For this review, use the dimensioned drawing (mm, ordinates from the lowest corner) and the shaded views. Round coordinates to 2 decimals unless told otherwise and drop trailing zeros. Loops run counter-clockwise (first coordinate to the right, second up) from the corner with the lowest first, then second, coordinate; pieces in that order, holes last. Notation, with made-up numbers: (68.5, 2) -> (108.5, 2) arc R25 ccw to (108.5, 24) -> close; hole circle Ø8 at (9.5, -25). An arc over 180 degrees is marked (long way). Answer as CSV lines item,"result". Start each with the question number.
(1) Draft analysis for pull direction X (two halves, no side actions). For the marked faces 1, 2 and 3, state which applies: +X half, -X half, draft (parallel to the pull), parting line (faces both ways), or undercut.
(2) Take a section at C-C, the plane x = 52. Write out the cut boundary in (y, z), and give its area (3 significant figures).
(3) For P1, Ø15, axis at y = 7.5, z = 29, coming from the -X side; P2, Ø2, axis at x = 76, z = 15.5, coming from the -Y side; P3, Ø15, axis at y = 13.5, z = 31, coming from the +X side, all flat-tipped, find the tip position at first contact; note any pin that passes through.
(4) Take a section at A-A, the plane y = 9. Write out the cut boundary in (x, z).
(5) To check wall thickness, follow line 1 (Y direction, x = 48, z = 57). State the ranges of the line that lie inside material, in increasing order. Write a range as from..to.
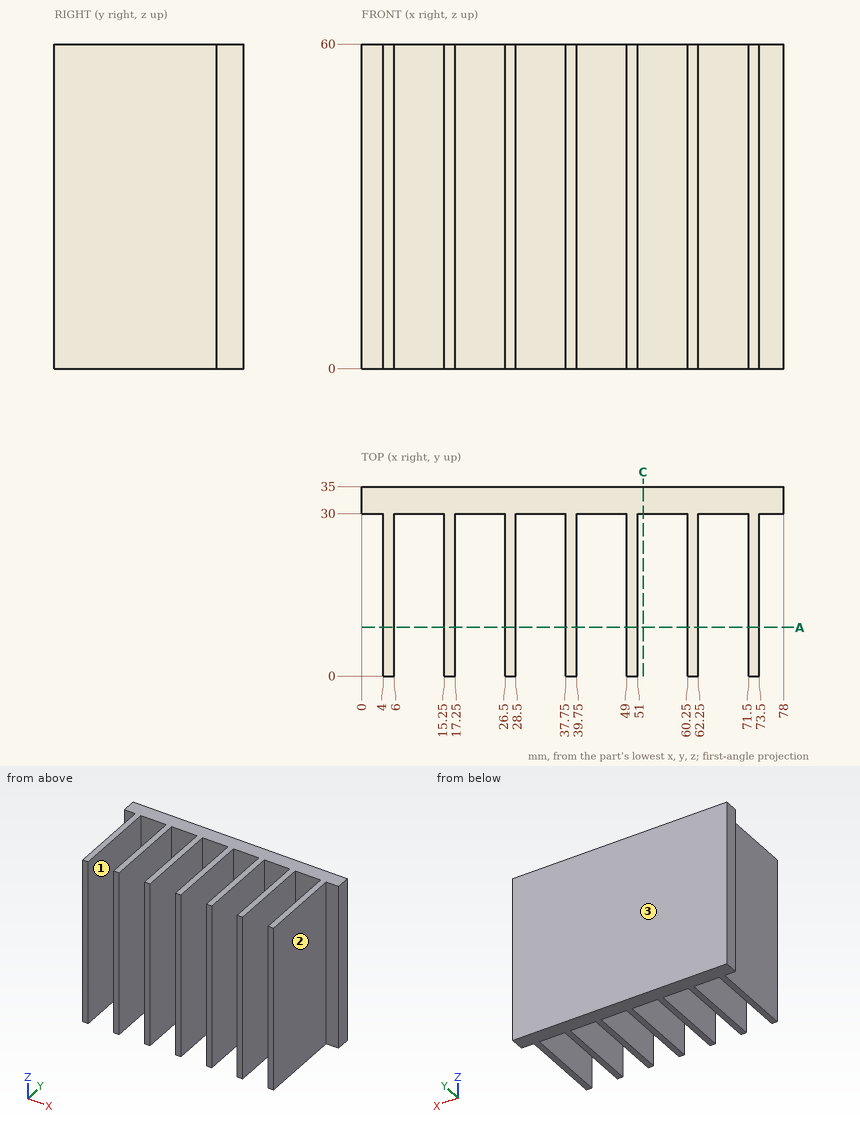
The answers:
1,face 1,"undercut"
1,face 2,"+X half"
1,face 3,"draft"
2,outline,"(30, 0) -> (35, 0) -> (35, 60) -> (30, 60) -> close"
2,area,"300 mm²"
3,P1,"x = 4"
3,P2,"y = 30"
3,P3,"x = 73.5"
4,outline,"(4, 0) -> (6, 0) -> (6, 60) -> (4, 60) -> close; (15.25, 0) -> (17.25, 0) -> (17.25, 60) -> (15.25, 60) -> close; (26.5, 0) -> (28.5, 0) -> (28.5, 60) -> (26.5, 60) -> close; (37.75, 0) -> (39.75, 0) -> (39.75, 60) -> (37.75, 60) -> close; (49, 0) -> (51, 0) -> (51, 60) -> (49, 60) -> close; (60.25, 0) -> (62.25, 0) -> (62.25, 60) -> (60.25, 60) -> close; (71.5, 0) -> (73.5, 0) -> (73.5, 60) -> (71.5, 60) -> close"
5,line 1,"30..35"
